Autodesk Inventor part; units mm, degrees
ref_plane "YZ Plane" through (0, 0, 0) normal (1, 0, 0) x (0, 1, 0)
ref_plane "XZ Plane" through (0, 0, 0) normal (0, 1, 0) x (-1, 0, 0)
ref_plane "XY Plane" through (0, 0, 0) normal (0, 0, 1) x (1, 0, 0)
sketch "Sketch1" plane through (0, 0, 0) normal (0, 1, 0) x (-1, 0, 0)
  circle A0 centre (0, 0) radius 135
  circle A1 centre (0, 0) radius 110
  dimension "d0" = 270
  dimension "d1" = 220
extrude "Extrusion1" add sketch "Sketch1" along normal mid plane 47
sketch "Sketch2" plane through (0, 0, 0) normal (0, 0, 1) x (1, 0, 0)
  circle A0 centre (0, -20.5) radius 18
  line L0 (-135, -23.5) -> (135, -23.5)
  dimension "d4" = 36
  dimension "d38" = 3
extrude "Extrusion2" cut sketch "Sketch2" against normal through all
sketch "Sketch3" plane through (0, 23.5, 0) normal (0, 1, 0) x (1, 0, 0)
  circle A0 centre (0, 0) radius 127.5
  circle A1 centre (-127.5, 0) radius 2
  circle A2 centre (-103.1497, -74.9426) radius 2
  circle A3 centre (-39.3997, -121.2597) radius 2
  circle A4 centre (39.3997, -121.2597) radius 2
  circle A5 centre (103.1497, -74.9426) radius 2
  circle A6 centre (127.5, 0) radius 2
  circle A7 centre (103.1497, 74.9426) radius 2
  circle A8 centre (39.3997, 121.2597) radius 2
  circle A9 centre (-39.3997, 121.2597) radius 2
  circle A10 centre (-103.1497, 74.9426) radius 2
  dimension "d7" = 255
  dimension "d8" = 4
  dimension "d11" = 360
hole "Hole1" at (39.3997, 23.5, 121.2597) at (-39.3997, 23.5, 121.2597) at (-103.1497, 23.5, 74.9426) at (-127.5, 23.5, 0) at (-103.1497, 23.5, -74.9426) at (-39.3997, 23.5, -121.2597) at (39.3997, 23.5, -121.2597) at (103.1497, 23.5, -74.9426) at (127.5, 23.5, 0) at (103.1497, 23.5, 74.9426) direction (0, -1, 0) diameter 5 end through all
sketch "Sketch4" plane through (0, 23.5, 0) normal (0, 1, 0) x (1, 0, 0)
  circle A0 centre (0, 0) radius 140
extrude "Extrusion3" cut sketch "Sketch4" against normal blind 27
sketch "Sketch7" plane through (0, -3.5, 0) normal (0, 1, 0) x (1, 0, 0)
  line L0 (0, 0) -> (70, 0)
  line L1 (80, -100) -> (60, -100)
  line L2 (60, -100) -> (60, 100)
  line L3 (60, 100) -> (80, 100)
  line L4 (80, 100) -> (80, -100)
  line L5 (80, -100) -> (60, 100) construction
  line L6 (60, -100) -> (80, 100) construction
  dimension "d39" = 70
  dimension "d40" = 20
  dimension "d41" = 200
extrude "Extrusion7" cut sketch "Sketch7" against normal blind 15
properties part number "Cylinder Spacer Bottom"
Could you check a few things on this model? Use its own coordinates, in mm. A direction names the side the tool comes from. Give positions to 0.01 mm unless a question says otherwise; leave off trailing zeros. Order: outer loops, then holes, each group sorted by start corner. A loop starts at its lowest first (then second) coordinate and runs counter-clockwise, first axis right, second up. Notation, with made-up numbers: (43.25, -22) - (80.25, -22) arc R17 cw to (80.25, -11) - close; hole circle Ø2 at (21, 89.5). An arc over 180 degrees is marked (long way). Return JSON: item names as keys, results as strings. Group by question number.
Q1. Suppose I cut it at B-B, the plane y = -13. State how many separate pieces and enclosed holes the cut face has, and give its area (3 significant figures).
Q2. Which directions (+Z, -Z, +X, -X, +Y, -Y) give clear straight access to the entire face, cutting with the end or side of a thin tool? Please do faces 4 (the face through (-15.4, -11.18, -121.51)), 5 (the face through (72, -18.5, 90)), 6 (the face through (-94.856, -13.36, -55.699)).
Q3. Please list where these lines run through material, in increasing order: line 1 along X through (y, z) = (-17, 0); line 2 along X through (y, z) = (-14, 76); line 3 along Z through (x, y) = (65, -15.75). Write a range as [from, to].
Q4. Suppose I cut it at A-A, the plane x = -75. Please give me the cut outline in (y, z), and give its area (3 significant figures).
Q5. Suppose I cut it at D-D, the plane x = 31.5. Please give me the cut outline in (y, z).
Q6. Thinking about a two-plate mould opening in X: for faces 1 (the face through (60, -11, -96)), 2 (the face through (70, -11, 100)), 3 (the face through (1, -23.5, 111)), which applies, pulls with the +X half, pulls with the -X half, needs draft (parallel to the pull), parting line crosses it, or undercut?
Q7. Will these pins go through, and if not, where does the flat tip stop? pin 1 Ø4 at (y, z) = (-9, 12.5) entering from +X; pin 2 Ø5 at (y, z) = (-15.5, -28.5) entering from +X; pin 3 Ø4.5 at (y, z) = (-12.5, -91) entering from -X.
Q8. Suppose I cut it at C-C, the plane z = -86. Please give me the cut outline in (x, y), and give its area (3 significant figures).
Resolved:
{
 "1": {"separate pieces": "1", "enclosed holes": "10", "area": "17,600 mm2"},
 "2": {"face 4": "-Z", "face 5": "+Y", "face 6": "+Y, -Y"},
 "3": {"line 1": "x = [-135, -130], [-125, -110], [110, 125], [130, 135]", "line 2": "x = [-111.58, -105.42], [-100.88, -79.52], [80, 100.88], [105.42, 111.58]", "line 3": "z = [-118.32, -100], [100, 118.32]"},
 "4": {"outline": "(-23.5, -112.25) - (-3.5, -112.25) - (-3.5, -80.47) - (-23.5, -80.47) - close; (-23.5, 80.47) - (-3.5, 80.47) - (-3.5, 112.25) - (-23.5, 112.25) - close", "area": "1,270 mm2"},
 "5": {"outline": "(-23.5, -131.27) - (-3.5, -131.27) - (-3.5, -105.39) - (-23.5, -105.39) - close; (-23.5, 105.39) - (-3.5, 105.39) - (-3.5, 131.27) - (-23.5, 131.27) - close"},
 "6": {"face 1": "undercut", "face 2": "undercut", "face 3": "needs draft"},
 "7": {"pin 1": "stops at x = 134.59", "pin 2": "stops at x = 132.47", "pin 3": "stops at x = -101.73"},
 "8": {"outline": "(-104.06, -23.5) - (-68.59, -23.5) - (-68.59, -3.5) - (-104.06, -3.5) - close; (68.59, -23.5) - (104.06, -23.5) - (104.06, -3.5) - (80, -3.5) - (80, -18.5) - (68.59, -18.5) - close", "area": "1,250 mm2"}
}
